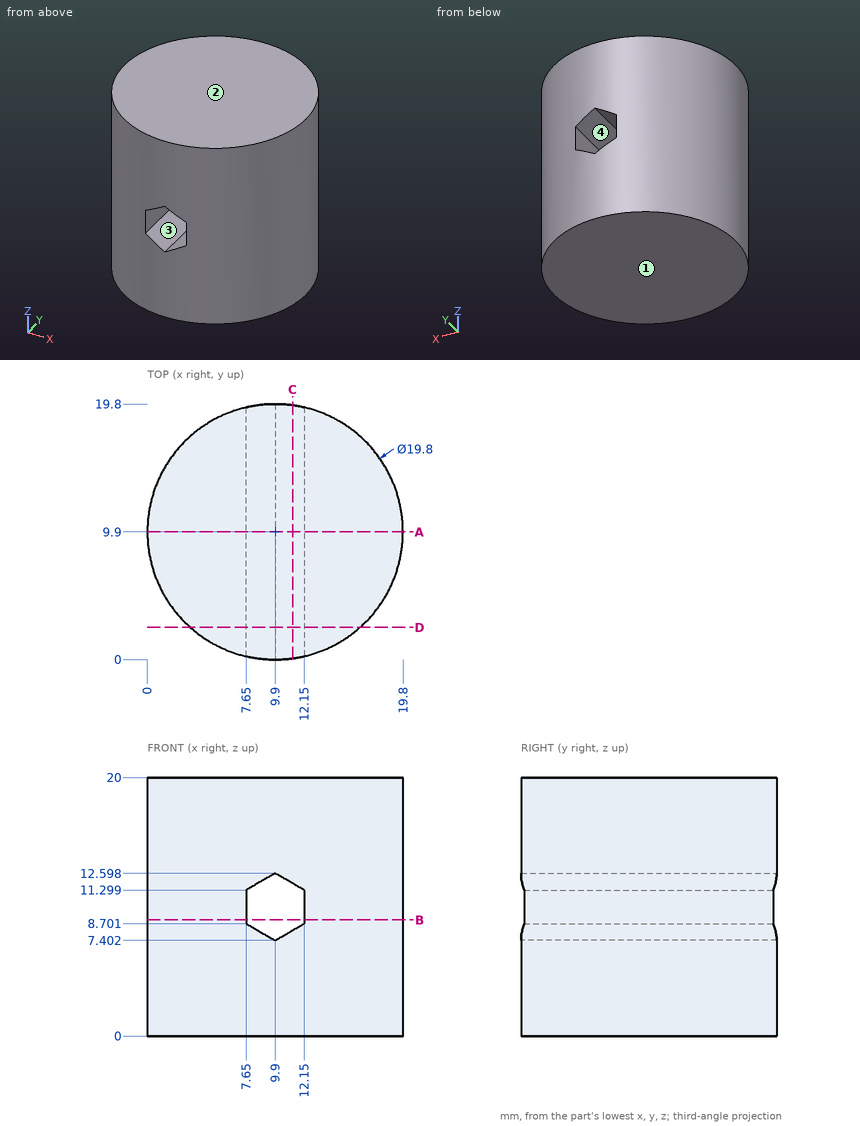
Here's the drawing with two shaded views (mm, measured from the low corner). I have some questions. Give positions to 0.01 mm unless a question says otherwise; leave off trailing zeros. Loops run counter-clockwise (first coordinate to the right, second up) from the corner with the lowest first, then second, coordinate; pieces in that order, holes last. Notation, with made-up numbers: M 68,36.5 L 90,36.5 A20 cw 90,53.5 Z; hole C 9.25,88 d9. An arc over 180 degrees is marked long. One line per item, written item: value. Start each with the question number.
1) If we section it at B-B, the plane z = 9: Write out the boundary of the cut face in (x, y).
2) Thinking about a two-plate mould opening in Z: for the marked faces 1, 2, 3 and 4, which applies, +Z half, -Z half, draft (parallel to the pull), parting line (faces both ways), or undercut?
3) If we section it at D-D, the plane y = 2.5: Write out the boundary of the cut face in (x, z), and give its area (3 significant figures).
4) If we section it at C-C, the plane x = 11.25: Write out the boundary of the cut face in (y, z), and give its area (3 significant figures).
5) If we section it at A-A, the plane y = 9.9: Write out the boundary of the cut face in (x, z).
6) I'm going to push flat-ended pins straight in: pin 1 (2 mm diameter, centred on x = 14.5, z = 5, fed in from -Y); pin 2 (3 mm diameter, centred on y = 13, z = 12.5, fed in from +X); pin 3 (0.8 mm diameter, centred on y = 8, z = 9.5, fed in from -X). Where does each tip first touch, or does it pass through?
7) If I drill on line 1 (Z direction, x = 8.5, y = 9); line 2 (Y direction, x = 9.75, z = 2.25); line 3 (X direction, y = 18.75, z = 8.5), over which ranges is the centre line in solid material (lowest first)? Write a range as [from, to].
Completed:
1. outline: M 7.65,0.26 L 7.65,19.54 A9.9 ccw Z; M 12.15,0.26 A9.9 ccw 12.15,19.54 Z
2. face 1: -Z half
2. face 2: +Z half
2. face 3: undercut
2. face 4: undercut
3. outline: M 3.32,0 L 16.48,0 L 16.48,20 L 3.32,20 Z; hole M 7.65,8.7 L 9.9,7.4 L 12.15,8.7 L 12.15,11.3 L 9.9,12.6 L 7.65,11.3 Z
3. area: 246 mm^2
4. outline: M 0.09,0 L 19.71,0 L 19.71,8.18 L 0.09,8.18 Z; M 0.09,11.82 L 19.71,11.82 L 19.71,20 L 0.09,20 Z
4. area: 321 mm^2
5. outline: M 0,0 L 19.8,0 L 19.8,20 L 0,20 Z; hole M 7.65,8.7 L 9.9,7.4 L 12.15,8.7 L 12.15,11.3 L 9.9,12.6 L 7.65,11.3 Z
6. pin 1: stops at y = 0.68
6. pin 2: stops at x = 19.67
6. pin 3: stops at x = 0.11
7. line 1: z = [0, 8.21], [11.79, 20]
7. line 2: y = [0, 19.8]
7. line 3: x = [5.46, 8], [11.8, 14.34]
